Build history of the part. All positions in model axes, mm. Give positions to 0.01 mm unless a question says otherwise; leave off trailing zeros. Loops run counter-clockwise (first coordinate to the right, second up) from the corner with the lowest first, then second, coordinate; pieces in that order, holes last.
1) Band-saw the part on A-A on x = 101.6. List the corners of the cut face in (y, z) (3 decimals), then the cut area to 3 significant figures.
2) Flat gauge pin, fed straight in: P1, Ø5, axis at x = -101.6, z = 12.7, coming from the -Y side. Where does the tip first touch, or does it go through?
3) Wall check: line 1 (X direction, y = 2.4, z = 12.7); line 2 (Z direction, x = -100.5, y = 0.55). Give the ranges that are in metal, low to high.
4) Band-saw the part on B-B on z = 12.7. List the corners of the cut face in (x, y) (3 decimals).
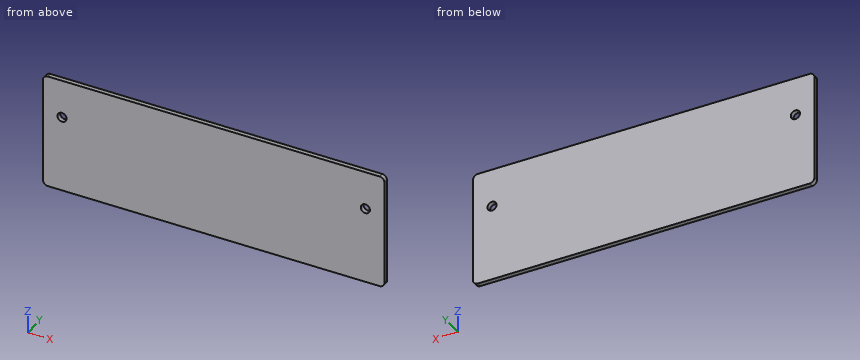
```python
from build123d import *

# Parameters (mm, degrees)
SKETCH1_W           = 228.6
SKETCH1_H           = 76.2
BOSS_EXTRUDE1_DEPTH = 3.175
SKETCH2_R           = 3.048
CUT_EXTRUDE1_DEPTH  = 10
FILLET1_R           = 3.175


with BuildPart() as part:
    # Sketch1 → Boss-Extrude1 (new body)
    with BuildSketch(Plane(origin=(0, 0, 0), x_dir=(1, 0, 0), z_dir=(0, 1, 0))):
        Rectangle(SKETCH1_W, SKETCH1_H)
    extrude(amount=BOSS_EXTRUDE1_DEPTH)

    # Sketch2 → Cut-Extrude1 (cut)
    with BuildSketch(Plane(origin=(0, 3.175, 0), x_dir=(1, 0, 0), z_dir=(0, 1, 0))):
        with Locations(Location((-101.6, -12.7, 0), (0, 0, 270))):
            Circle(SKETCH2_R)
        with Locations(Location((101.6, -12.7, 0), (0, 0, 270))):
            Circle(SKETCH2_R)
    extrude(amount=-CUT_EXTRUDE1_DEPTH, mode=Mode.SUBTRACT)

    # Fillet1
    fillet1_edges = [part.edges().sort_by_distance(p)[0] for p in [
        (-114.3, 1.5875, -38.1),
        (114.3, 1.5875, -38.1),
        (114.3, 1.5875, 38.1),
        (-114.3, 1.5875, 38.1),
    ]]
    fillet(fillet1_edges, radius=FILLET1_R)


solid = part.part
```
Findings below:
1. outline: (0, -38.1) - (3.175, -38.1) - (3.175, 9.652) - (0, 9.652) - close; (0, 15.748) - (3.175, 15.748) - (3.175, 38.1) - (0, 38.1) - close
1. area: 223 mm2
2. P1: passes through
3. line 1: x = -114.3 to -104.65, -98.55 to 98.55, 104.65 to 114.3
3. line 2: z = -38.1 to 9.86, 15.54 to 38.1
4. outline: (-114.3, 0) - (-104.648, 0) - (-104.648, 3.175) - (-114.3, 3.175) - close; (-98.552, 0) - (98.552, 0) - (98.552, 3.175) - (-98.552, 3.175) - close; (104.648, 0) - (114.3, 0) - (114.3, 3.175) - (104.648, 3.175) - close
